Input: part model. Units: mm. Frame: model coordinates. Round coordinates to 2 decimals unless told otherwise and drop trailing zeros. Write each loop counter-clockwise with the first axis right and the second up, starting at its lowest first coordinate (ties: lowest second). Pieces come first, ordered by that corner, then holes. Notation, with made-up numbers: (7, 0) - (50, 0) arc R11 cw to (50, 12) - close; hole circle Ø6 at (83, -35.5). An arc over 180 degrees is marked (long way). Use one line per item in the form item = value.
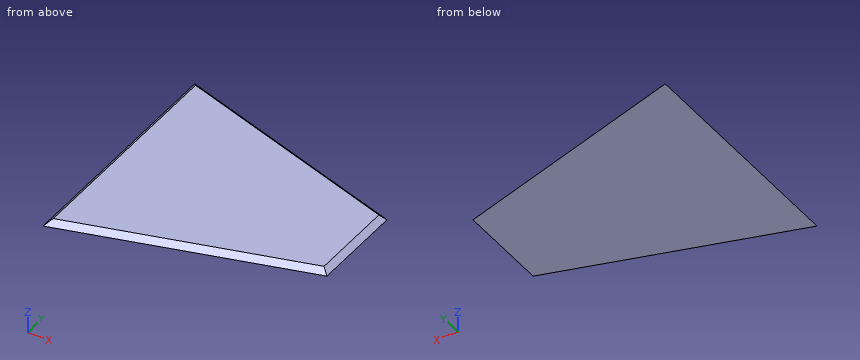
```python
from build123d import *

# Parameters (mm, degrees)
AUFSATZ_LINEAR_AUSTRAGEN1_DEPTH = 10
FASE1_SIZE                      = 10


with BuildPart() as part:
    # Skizze1 → Aufsatz-Linear austragen1 (new body)
    with BuildSketch(Plane.XY):
        Polygon((-434.714346895, -214.6), (-434.714346895, 214.6), (0, 85), (0, -85), align=None)
    extrude(amount=AUFSATZ_LINEAR_AUSTRAGEN1_DEPTH)

    # Fase1
    fase1_edges = [part.edges().sort_by_distance(p)[0] for p in [
        (-434.714346895, 0, 10),
        (-217.357173448, 149.8, 10),
        (0, 0, 10),
        (-217.357173448, -149.8, 10),
    ]]
    chamfer(fase1_edges, length=FASE1_SIZE - 0.0001)  # a hair under: the kernel refuses the full size


solid = part.part
```
(1) First-contact query: pin 1 Ø4 at (x, z) = (-104.5, 5) entering from -Y; pin 2 Ø1.5 at (x, z) = (-368.5, 5) entering from +Y; pin 3 Ø3 at (x, z) = (-208.5, 6) entering from +Y. Flat tips, straight axial feed; report the tip coordinate or a pass-through.
Derived:
pin_1 = -113.11
pin_2 = 190.46
pin_3 = 142.53
(2) Cut plane C-C on z = 8. Output: boundary loops of the cut face in (x, y), then the cut area to 3 significant figures.
Derived:
outline = (-426.71, -203.87) - (-8, -79.04) - (-8, 79.04) - (-426.71, 203.87) - close
area = 118,000 mm^2
(3) Material intervals for L1, parallel to Y at x = -128, z = 8; L2, parallel to X at y = -65, z = 3.75; L3, parallel to Y at x = -322.5, z = 7.5, sorted ascending.
Derived:
L1 = -114.81 to 114.81
L2 = -430.96 to -3.75
L3 = -173.32 to 173.32
